For this review, take the finished solid that the model builds, in its own axes (mm). A direction names the side the tool comes from. Coordinates: 2 decimals unless noted, no trailing zeros. Write each loop counter-clockwise with the first axis right and the second up, starting at its lowest first coordinate (ties: lowest second). Pieces come first, ordered by that corner, then holes. Notation, with made-up numbers: M 29,-28 L 51,-28 A24 ccw 51,-9 Z; hole C 14.5,33.5 d5. An arc over 180 degrees is marked long. Return JSON: item names as keys, results as strings.
```python
from build123d import *

# Parameters (mm, degrees)
SKETCH_1_W           = 42
SKETCH_1_H           = 21.4
EXTRUDE_1_DEPTH      = 12
SKETCH_2_W           = 6
SKETCH_2_H           = 2
CUT_EXTRUDE_1_DEPTH  = 49.641134855
SKETCH_3_R           = 5
CUT_EXTRUDE_2_DEPTH  = 5.5
SKETCH_3_3_R         = 8.5
CUT_EXTRUDE_3_DEPTH  = 3
SKETCH_3_4_R         = 3.5
CUT_EXTRUDE_4_DEPTH  = 7
SKETCH_3_5_R         = 5
CUT_EXTRUDE_5_DEPTH  = 8.5
CUT_EXTRUDE_START    = -8.5
SKETCH_3_6_R         = 3.1
CUT_EXTRUDE_6_DEPTH  = 2.6
CUT_EXTRUDE_START_2  = -5.5
SKETCH_3_7_R         = 3.1
CUT_EXTRUDE_7_DEPTH  = 2.6
EXTRUDE_START        = -2
SKETCH_4_W           = 42
SKETCH_4_H           = 21.4
SKETCH_4_W_2         = 45
SKETCH_4_H_2         = 10
EXTRUDE_2_DEPTH      = 5
SKETCH_5_R           = 2.25
CUT_EXTRUDE_8_DEPTH  = 3
SKETCH_5_3_R         = 1.5
CUT_EXTRUDE_9_DEPTH  = 86.586213843
SKETCH_3_8_R         = 1.05
SKETCH_3_8_R_2       = 2
CUT_EXTRUDE_10_DEPTH = 87.313382508
SKETCH_6_R           = 1.5
CUT_EXTRUDE_11_DEPTH = 87.313382508
SKETCH_6_3_R         = 2.25
CUT_EXTRUDE_12_DEPTH = 3
SKETCH_7_R           = 0.8
CUT_EXTRUDE_13_DEPTH = 4
SKETCH_3_9_R         = 3.1
CUT_EXTRUDE_14_DEPTH = 2.6


with BuildPart() as part:
    # 草图1 → 凸台-拉伸1 (new body)
    with BuildSketch(Plane(origin=(0, 0, 0), x_dir=(1, 0, 0), z_dir=(0, 1, 0))):
        with Locations((21, -10.7)):
            Rectangle(SKETCH_1_W, SKETCH_1_H)
    extrude(amount=EXTRUDE_1_DEPTH)

    # 草图2 → 切除-拉伸1 (cut, through all)
    with BuildSketch(Plane(origin=(0, 0, 0), x_dir=(-1, 0, 0), z_dir=(0, 0, -1))):
        Polygon((-10, 0), (0, 0), (0, 10), (-10, 10), (-10, 2), align=None)
        with Locations((-13, 1)):
            Rectangle(SKETCH_2_W, SKETCH_2_H)
    extrude(amount=-CUT_EXTRUDE_1_DEPTH, mode=Mode.SUBTRACT)

    # 草图3 → 切除-拉伸2 (cut)
    with BuildSketch(Plane.XZ):
        with Locations(Location((20.3, 7.4, 0), (0, 0, 270))):
            Circle(SKETCH_3_R)
    extrude(amount=-CUT_EXTRUDE_2_DEPTH, mode=Mode.SUBTRACT)

    # 草图3<3> → 切除-拉伸3 (cut)
    with BuildSketch(Plane.XZ):
        with Locations((31.64970263, 9.253173011)):
            Circle(SKETCH_3_3_R)
    extrude(amount=-CUT_EXTRUDE_3_DEPTH, mode=Mode.SUBTRACT)

    # 草图3<4> → 切除-拉伸4 (cut)
    with BuildSketch(Plane.XZ):
        with Locations(Location((31.64970263, 9.253173011, 0), (0, 0, 270))):
            Circle(SKETCH_3_4_R)
    extrude(amount=-CUT_EXTRUDE_4_DEPTH, mode=Mode.SUBTRACT)

    # 草图3<5> → 切除-拉伸5 (cut)
    with BuildSketch(Plane.XZ):
        with Locations(Location((32.76916715, 15.656047301, 0), (0, 0, 270))):
            Circle(SKETCH_3_5_R)
    extrude(amount=-CUT_EXTRUDE_5_DEPTH, mode=Mode.SUBTRACT)

    # 草图3<6> → 切除-拉伸6 (cut)
    with BuildSketch(Plane.XZ.offset(CUT_EXTRUDE_START)):
        with Locations(Location((32.76916715, 15.656047301, 0), (0, 0, 270))):
            Circle(SKETCH_3_6_R)
    extrude(amount=-CUT_EXTRUDE_6_DEPTH, mode=Mode.SUBTRACT)

    # 草图3<7> → 切除-拉伸7 (cut)
    with BuildSketch(Plane.XZ.offset(CUT_EXTRUDE_START_2)):
        with Locations(Location((20.3, 7.4, 0), (0, 0, 270))):
            Circle(SKETCH_3_7_R)
    extrude(amount=-CUT_EXTRUDE_7_DEPTH, mode=Mode.SUBTRACT)

    # 草图4 → 凸台-拉伸2 (add)
    with BuildSketch(Plane(origin=(0, 12, 0), x_dir=(1, 0, 0), z_dir=(0, 1, 0)).offset(EXTRUDE_START)):
        with Locations((21, -10.7)):
            Rectangle(SKETCH_4_W, SKETCH_4_H)
        Polygon((0, -21.4), (0, 0), (-32, 0), (-32, -14.5), (-32, -24.5), (-32, -36), (0, -36), align=None)
        with Locations((-54.5, -19.5)):
            Rectangle(SKETCH_4_W_2, SKETCH_4_H_2)
    extrude(amount=EXTRUDE_2_DEPTH)

    # 草图5 → 切除-拉伸8 (cut)
    with BuildSketch(Plane.XZ.offset(-10)):
        with Locations((-7.480832871, 32.656047307)):
            Circle(SKETCH_5_R)
        with Locations((-21.980832871, 32.656047307)):
            Circle(SKETCH_5_R)
        with Locations((-70.230832871, 19.656047307)):
            Circle(SKETCH_5_R)
    extrude(amount=-CUT_EXTRUDE_8_DEPTH, mode=Mode.SUBTRACT)

    # 草图5<3> → 切除-拉伸9 (cut, through all)
    with BuildSketch(Plane.XZ.offset(-10)):
        with Locations((-70.230832871, 19.656047307)):
            Circle(SKETCH_5_3_R)
        with Locations((-21.980832871, 32.656047307)):
            Circle(SKETCH_5_3_R)
        with Locations((-7.480832871, 32.656047307)):
            Circle(SKETCH_5_3_R)
    extrude(amount=-CUT_EXTRUDE_9_DEPTH, mode=Mode.SUBTRACT)

    # 草图3<8> → 切除-拉伸10 (cut, through all)
    with BuildSketch(Plane.XZ):
        with Locations(Location((31.64970263, 9.253173011, 0), (0, 0, 270))):
            Circle(SKETCH_3_8_R)
        with Locations(Location((32.76916715, 15.656047301, 0), (0, 0, 270))):
            Circle(SKETCH_3_8_R_2)
    extrude(amount=-CUT_EXTRUDE_10_DEPTH, mode=Mode.SUBTRACT)

    # 草图6 → 切除-拉伸11 (cut, through all)
    with BuildSketch(Plane(origin=(0, 15, 0), x_dir=(1, 0, 0), z_dir=(0, 1, 0))):
        with Locations(Location((5, -5, 0), (0, 0, 180))):
            Circle(SKETCH_6_R)
        with Locations(Location((5, -16.4, 0), (0, 0, 180))):
            Circle(SKETCH_6_R)
    extrude(amount=-CUT_EXTRUDE_11_DEPTH, mode=Mode.SUBTRACT)

    # 草图6<3> → 切除-拉伸12 (cut)
    with BuildSketch(Plane(origin=(0, 15, 0), x_dir=(1, 0, 0), z_dir=(0, 1, 0))):
        with Locations(Location((5, -5, 0), (0, 0, 180))):
            Circle(SKETCH_6_3_R)
        with Locations(Location((5, -16.4, 0), (0, 0, 180))):
            Circle(SKETCH_6_3_R)
    extrude(amount=-CUT_EXTRUDE_12_DEPTH, mode=Mode.SUBTRACT)

    # 草图7 → 切除-拉伸13 (cut)
    with BuildSketch(Plane.XZ):
        with Locations(Location((39.5, 18.4, 0), (0, 0, 270))):
            Circle(SKETCH_7_R)
        with Locations(Location((39.5, 2.5, 0), (0, 0, 270))):
            Circle(SKETCH_7_R)
    extrude(amount=-CUT_EXTRUDE_13_DEPTH, mode=Mode.SUBTRACT)

    # 草图3<9> → 切除-拉伸14 (cut)
    with BuildSketch(Plane.XZ.offset(CUT_EXTRUDE_START)):
        with Locations(Location((32.76916715, 15.656047301, 0), (0, 0, 270))):
            Circle(SKETCH_3_9_R)
    extrude(amount=-CUT_EXTRUDE_14_DEPTH, mode=Mode.SUBTRACT)


solid = part.part
```
1. Wall thickness on L1, parallel to Y at x = -13.5, z = 26; L2, parallel to Z at x = -34.5, y = 13.75; L3, parallel to Z at x = -72, y = 11.25: over which ranges is each line inside the solid? List them lowest first. Write a range as from..to.
Checks:
{"L1": "10..15", "L2": "14.5..24.5", "L3": "14.5..18.27, 21.05..24.5"}
2. We need section C-C (x = 20.3). State the section outline as (y, z) points, plus the area to 3 significant figures.
Checks:
{"outline": "M 0,0 L 15,0 L 15,21.4 L 0,21.4 L 0,12.4 L 5.5,12.4 L 5.5,10.5 L 8.1,10.5 L 8.1,4.3 L 5.5,4.3 L 5.5,2.4 L 0,2.4 Z", "area": "250 mm2"}
3. For faces 1 (the face through (5, 12, 7)), 2 (the face through (-24, 10, 18)), 3 (the face through (31, 7, 8)), list the 3-axis set-ups (+Z, -Z, +X, -X, +Y, -Y) from which the entire face can be reached by the end or side of a thin tool; tool diameter is ignored.
Checks:
{"face 1": "+Y", "face 2": "+Z, -Z, -X, -Y", "face 3": "-Y"}
4. Clearance check with flat-ended pins moving along their axes: pin 1 Ø5 at (x, z) = (20, 8.5) entering from -Y; pin 2 Ø11.5 at (x, z) = (20.3, 7.4) entering from -Y; pin 3 Ø8 at (y, z) = (13.5, 7.5) entering from -X; pin 4 Ø10 at (x, z) = (-27, 24) entering from -Y. State where each tip first meets the part, or that it passes through.
Checks:
{"pin 1": "y = 5.5", "pin 2": "y = 0", "pin 3": "x = -32", "pin 4": "y = 10"}
5. We need section A-A (x = 5). State the section outline as (y, z) points.
Checks:
{"outline": "M 10,0 L 15,0 L 15,2.75 L 12,2.75 L 12,3.5 L 10,3.5 Z; M 10,6.5 L 12,6.5 L 12,7.25 L 15,7.25 L 15,14.15 L 12,14.15 L 12,14.9 L 10,14.9 Z; M 10,17.9 L 12,17.9 L 12,18.65 L 15,18.65 L 15,21.4 L 10,21.4 Z"}
6. We need section B-B (z = 29). State the section outline as (x, y) points.
Checks:
{"outline": "M -32,10 L 0,10 L 0,15 L -32,15 Z"}
7. Draft analysis for pull direction Z (two halves, no side actions). For faces 4 (the face through (0, 12, 29)), 5 (the face through (-16, 12, 36)), 6 (the face through (-55, 12, 14.5)), 7 (the face through (-22, 13, 31)), state which applies: +Z half, -Z half, draft (parallel to the pull), parting line (faces both ways), or undercut.
Checks:
{"face 4": "draft", "face 5": "+Z half", "face 6": "-Z half", "face 7": "undercut"}
8. We need section D-D (x = -44). State the section outline as (y, z) points.
Checks:
{"outline": "M 10,14.5 L 15,14.5 L 15,24.5 L 10,24.5 Z"}
